Read the model definition and answer for the solid it produces. Units are mm, in the model's axes. A direction names the side the tool comes from. Give positions to 0.01 mm unless a question says otherwise; leave off trailing zeros. Order: outer loops, then holes, each group sorted by start corner. A loop starts at its lowest first (then second) coordinate and runs counter-clockwise, first axis right, second up. Notation, with made-up numbers: (70, -38.5) - (119, -38.5) arc R25 cw to (119, -10.5) - close; hole circle Ø9 at (52.25, 24). An arc over 180 degrees is marked (long way). Use a Markdown table: item, result. Add a question column.
1. A cutting plane is placed at B-B on z = 0. Determine the outline of the cut face in (x, y).
2. For a pull along Z with two mould halves and no side action, classify faces 4 (the cylindrical face through (3.233, 2.566, -1.341)), 5 (the flat face through (0.99, 1.13, -1.74)), 6 (the flat face through (-2, 5, -2)) as released by +Z, released by -Z, zero draft, split by the parting line, or undercut.
3. Consider L1, parallel to Y at x = 0.5, z = 3; L2, parallel to X at y = 10.5, z = 1.5; L3, parallel to Y at x = 1, z = 0.5. Determine where each line is inside the solid, lowest interval first.
4. Which of the six approach directions +Z, -Z, +X, -X, +Y, -Y give full straight-line access (tool end or side, diameter ignored) to faces 1 (the flat face through (-1.014, 1.134, -1.724)), 2 (the flat face through (0, 30, 0)), 3 (the cylindrical face through (0.54, 17.32, 2.44))?
5. Flat-ended cylindrical pins translate along their axes: P1, Ø4, axis at x = -0.5, y = 3, coming from the -Z side; P2, Ø4, axis at x = -2, y = 21, coming from the +Z side; P3, Ø1.2, axis at x = 0.5, z = 1, coming from the -Y side; P4, Ø1.5, axis at y = 16, z = 1.5, coming from the -X side. Find the tip coordinate at first contact, or state that the pin passes through.
6. A cutting plane is placed at C-C on y = 16.5. Determine the outline of the cut face in (x, z).
7. A cutting plane is placed at A-A on y = 2. Determine the outline of the cut face in (x, z).
Solid Edge part; units mm, degrees
sketch "Sketch1" plane through (0, 0, 0) normal (0, -1, 0) x (1, 0, 0)
  circle A0 centre (0, 0) radius 3.5
extrude "Protrusion1" add sketch "Sketch1" against normal blind 5
sketch "Sketch2" plane through (0, 5, 0) normal (0, 1, 0) x (-1, 0, 0)
  circle A0 centre (0, 0) radius 2.5
extrude "ExtrudedProtrusion_2" add sketch "Sketch2" along normal blind 25
fillet "Round_1" radius 0.2 1 edges at (-3.5, 0, 0)
sketch "Sketch3" plane through (0, 0, 0) normal (0, -1, 0) x (1, 0, 0)
  line L0 (0, 2.3094) -> (-2, 1.1547)
  line L1 (-2, 1.1547) -> (-2, -1.1547)
  line L2 (-2, -1.1547) -> (0, -2.3094)
  line L3 (0, -2.3094) -> (2, -1.1547)
  line L4 (2, -1.1547) -> (2, 1.1547)
  line L5 (2, 1.1547) -> (0, 2.3094)
extrude "ExtrudedCutout_2" cut sketch "Sketch3" against normal blind 2.3
properties material "Steel"
Output values:
| question | item | result |
|---|---|---|
| 1 | outline | (-3.5, 0.2) arc R0.2 ccw to (-3.3, 0) - (-2, 0) - (-2, 2.3) - (2, 2.3) - (2, 0) - (3.3, 0) arc R0.2 ccw to (3.5, 0.2) - (3.5, 5) - (2.5, 5) - (2.5, 30) - (-2.5, 30) - (-2.5, 5) - (-3.5, 5) - close |
| 2 | face 4 | split by the parting line |
| 2 | face 5 | undercut |
| 2 | face 6 | zero draft |
| 3 | L1 | 0 to 5 |
| 3 | L2 | -2 to 2 |
| 3 | L3 | 2.3 to 30 |
| 4 | face 1 | -Y |
| 4 | face 2 | +Z, -Z, +X, -X, +Y |
| 4 | face 3 | +Y |
| 5 | P1 | z = -3.5 |
| 5 | P2 | z = 2.5 |
| 5 | P3 | y = 2.3 |
| 5 | P4 | x = -2.38 |
| 6 | outline | circle Ø5 at (0, 0) |
| 7 | outline | circle Ø7 at (0, 0); hole (-2, -1.15) - (0, -2.31) - (2, -1.15) - (2, 1.15) - (0, 2.31) - (-2, 1.15) - close |
